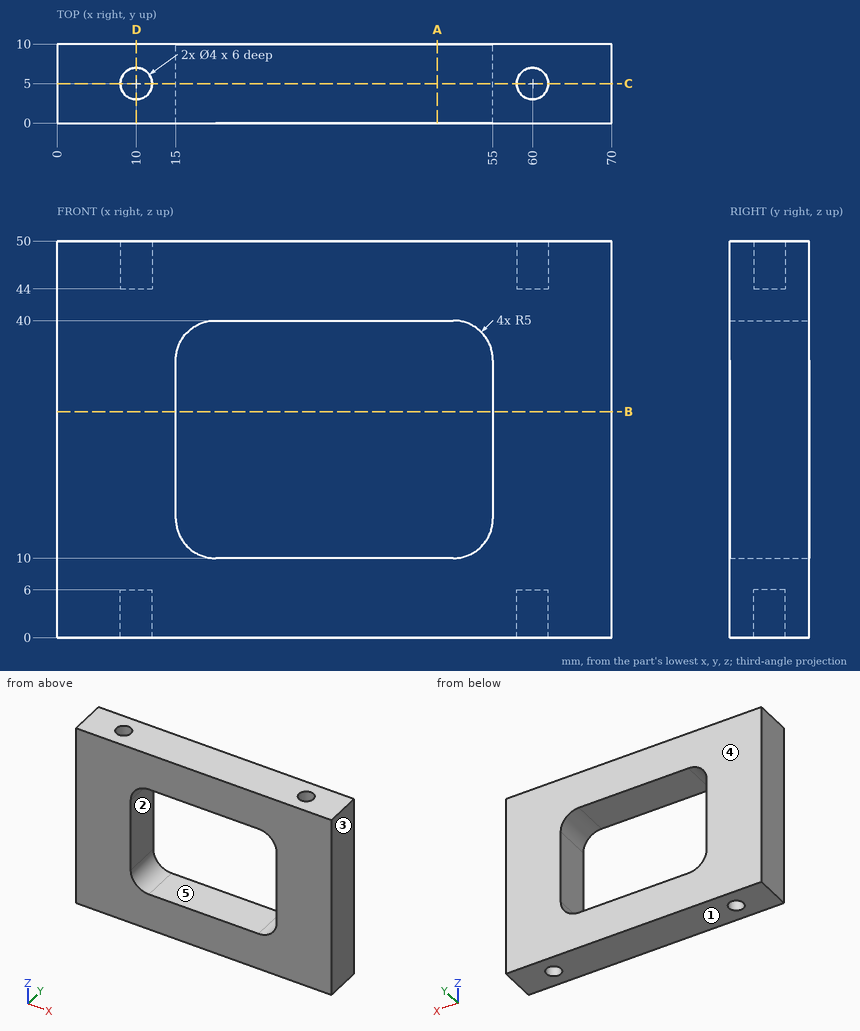
Drawing for the job (mm, zero at the part's lowest x, y, z). A direction names the side the tool comes from. Round coordinates to 2 decimals unless told otherwise and drop trailing zeros. Order: outer loops, then holes, each group sorted by start corner. A loop starts at its lowest first (then second) coordinate and runs counter-clockwise, first axis right, second up.
Item 1: Saw through at B-B on z = 28.5. Write the cut outline in (x, y), then the cut area to 3 significant figures.
Item 2: Saw through at C-C on y = 5. Write the cut outline in (x, z), then the cut area to 3 significant figures.
Item 3: Saw through at D-D on x = 10. Write the cut outline in (y, z), then the cut area to 3 significant figures.
Item 4: Saw through at A-A on x = 48. Write the cut outline in (y, z), then the cut area to 3 significant figures.
Item 5: Probe line 1 along X through (y, z) = (5, 2.6); line 2 along Y through (x, z) = (10, 46.55); line 3 along Z through (x, y) = (22, 9). List the from-to ranges inside material, lowest first.
Item 6: Tool access for the marked faces 4 and 5: list every direction of +Z, -Z, +X, -X, +Y, -Y with a clear straight run to the whole face (end or side of a thin tool).
Item 7: Mould opens along Z. For the marked faces 1, 2 and 3 say: pulls with the +Z half, pulls with the -Z half, needs draft (parallel to the pull), parting line crosses it, or undercut.
Item 8: Pin check, flat tip, straight feed: pin 1 (3 mm diameter, centred on x = 10, y = 5, fed in from +Z). Stop position of the tip, or through.
Reported:
1. outline: (0, 0) - (15, 0) - (15, 10) - (0, 10) - close; (55, 0) - (70, 0) - (70, 10) - (55, 10) - close
1. area: 300 mm2
2. outline: (0, 0) - (8, 0) - (8, 6) - (12, 6) - (12, 0) - (58, 0) - (58, 6) - (62, 6) - (62, 0) - (70, 0) - (70, 50) - (62, 50) - (62, 44) - (58, 44) - (58, 50) - (12, 50) - (12, 44) - (8, 44) - (8, 50) - (0, 50) - close; hole (15, 15) arc R5 ccw to (20, 10) - (50, 10) arc R5 ccw to (55, 15) - (55, 35) arc R5 ccw to (50, 40) - (20, 40) arc R5 ccw to (15, 35) - close
2. area: 2,230 mm2
3. outline: (0, 0) - (3, 0) - (3, 6) - (7, 6) - (7, 0) - (10, 0) - (10, 50) - (7, 50) - (7, 44) - (3, 44) - (3, 50) - (0, 50) - close
3. area: 452 mm2
4. outline: (0, 0) - (10, 0) - (10, 10) - (0, 10) - close; (0, 40) - (10, 40) - (10, 50) - (0, 50) - close
4. area: 200 mm2
5. line 1: x = 0 to 8, 12 to 58, 62 to 70
5. line 2: y = 0 to 3, 7 to 10
5. line 3: z = 0 to 10, 40 to 50
6. face 4: +Z, -Z, +X, -X, +Y
6. face 5: +Y, -Y
7. face 1: pulls with the -Z half
7. face 2: undercut
7. face 3: needs draft
8. pin 1: stops at z = 44
